Can you work these out from the model? Positions are in its coordinate system, mm. A direction names the side the tool comes from. Give positions to 0.01 mm unless a question says otherwise; leave off trailing zeros. Write each loop counter-clockwise with the first axis right and the second up, starting at its lowest first coordinate (ties: lowest second). Pieces come first, ordered by that corner, then holes.
1. I'm going to push flat-ended pins straight in: pin 1 (0.8 mm diameter, centred on x = 27.5, z = 14.5, fed in from -Y); pin 2 (8 mm diameter, centred on y = 25, z = 2.5, fed in from -X); pin 3 (1.5 mm diameter, centred on y = 3, z = 9.5, fed in from +X); pin 4 (3 mm diameter, centred on y = -14.5, z = 2, fed in from -X). Where does each tip first touch, or does it pass through?
2. Suppose I cut it at D-D (y = 3.5). Please give me the cut outline in (x, z), and give its area (3 significant figures).
3. Thinking about a two-plate mould opening in Y: for faces 1 (the flat face through (1, 59, 16)), 2 (the flat face through (8, -33.28, 3)), 3 (the flat face through (27, 1.8, 7.6)), which applies, pulls with the +Y half, pulls with the -Y half, needs draft (parallel to the pull), parting line crosses it, or undercut?
4. On a 3-axis mill with a long thin cutter (end or side, diameter ignored), from which of +Z, -Z, +X, -X, +Y, -Y can I reach the whole of each face in a straight line? I mean faces 4 (the flat face through (0, -21, 3)), 5 (the flat face through (0, 26, 3)), 6 (the flat face through (0, 59, 11)). Say none if no direction works.
5. Suppose I cut it at B-B (x = 20.5). Please give me the cut outline in (y, z), and give its area (3 significant figures).
6. Suppose I cut it at A-A (y = -18.5). Please give me the cut outline in (x, z), and give its area (3 significant figures).
7. Suppose I cut it at C-C (x = -5). Please give me the cut outline in (y, z).
8. If I drill on probe 1 along Y at (x, z) = (1, 4); probe 2 along X at (y, z) = (-3, 8.5); probe 3 along X at (y, z) = (-12.5, 5), over which ranges is the centre line in solid material (lowest first)?
```python
from build123d import *
from build123d import SkipClean  # not in build123d's __all__

# Parameters (mm, degrees)
F1_DEPTH  = 6
F3_DEPTH  = 10
F5_DEPTH  = 1
F7_DEPTH  = 1
F9_DEPTH  = 1
F10_DEPTH = 1
F13_DEPTH = 1


# Not quite as in the source:
# - ends of sketch curves that miss each other by under 0.0002 mm in the source are joined


with BuildPart() as f1:
    # F0 (on Top) → F1 (new body)
    with BuildSketch(Plane.XY):
        Polygon((-60, -8.2803227458), (-60, -33.2803227458), (-44, -33.2803227458), (-44, -8.2803227458), (0, -8.2803227458), (0, -33.2803227458), (16, -33.2803227458), (16, -8.2803227458), (28, -8.2803227458), (28, 11.7196772542), (0, 11.7196772542), (0, 40.7196772542), (28, 40.7196772542), (28, 60.7196772542), (-72, 60.7196772542), (-72, 40.7196772542), (-49, 40.7196772542), (-49, 11.7196772542), (-72, 11.7391310632), (-72, 11.693589665), (-72, 7.693589665), (-72, -4.280322887), (-72, -8.280322887), (-69, -8.2803227458), align=None)
    extrude(amount=F1_DEPTH)

    # F2 (on face) → F3 (join)
    with BuildSketch(Plane.XY.offset(6)):
        Polygon((-72, 60.7196772542), (-72, 56.7391310632), (-71, 56.7391310632), (-71, 58.7391310632), (-69, 58.7391310632), (-69, 60.7196772542), align=None)
        Polygon((-72, 40.7196773953), (-69, 40.7196773953), (-69, 42.7196773953), (-71, 42.7196773953), (-71, 44.7196773953), (-72, 44.7196773953), align=None)
        Polygon((-45, 42.7196773953), (-47, 42.7196773953), (-47, 40.7196773953), (-44, 40.7196773953), (-44, 44.7196773953), (-45, 44.7196773953), align=None)
        Polygon((-44, 60.7196772542), (-47, 60.7196772542), (-47, 58.7391310632), (-45, 58.7391310632), (-45, 56.7391310632), (-44, 56.7391310632), align=None)
        Polygon((28, 60.7196772542), (25, 60.7196772542), (25, 58.7391310632), (27, 58.7391310632), (27, 56.7391310632), (28, 56.7391310632), align=None)
        Polygon((25, 42.7196773953), (25, 40.7196773953), (28, 40.7196773953), (28, 44.7196773953), (27, 44.7196773953), (27, 42.7196773953), align=None)
        Polygon((0, 44.7196773953), (0, 40.7196772542), (3, 40.7196773953), (3, 42.7196773953), (1, 42.7196773953), (1, 44.7196773953), align=None)
        Polygon((3, 60.7196772542), (0, 60.7196772542), (0, 56.7391310632), (1, 56.7391310632), (1, 58.7391310632), (3, 58.7391310632), align=None)
        Polygon((27, 7.7391309221), (28, 7.7391309221), (28, 11.7196772542), (25, 11.7196772542), (25, 9.7391309221), (27, 9.7391309221), align=None)
        Polygon((25, -6.2803227458), (25, -8.2803227458), (28, -8.2803227458), (28, -4.2803227458), (27, -4.2803227458), (27, -6.2803227458), align=None)
        Polygon((0, -4.2803227458), (0, -8.280322887), (3, -8.2803227458), (3, -6.2803227458), (1, -6.2803227458), (1, -4.2803227458), align=None)
        Polygon((3, 9.7391309221), (3, 11.7196772542), (0, 11.7196772542), (0, 7.7391309221), (1, 7.7391309221), (1, 9.7391309221), align=None)
        Polygon((-45, 7.7391309221), (-44, 7.7391309221), (-44, 11.7391310632), (-47, 11.7391309221), (-47, 9.7391309221), (-45, 9.7391309221), align=None)
        Polygon((-47, -8.2803227458), (-44, -8.2803227458), (-44, -4.2803227458), (-45, -4.2803227458), (-45, -6.2803227458), (-47, -6.2803227458), align=None)
        Polygon((-72, -4.2803227458), (-72, -8.280322887), (-69, -8.2803227458), (-69, -6.2803227458), (-71, -6.2803227458), (-71, -4.2803227458), align=None)
        Polygon((-72, 11.7391310632), (-72, 7.7391309221), (-71, 7.7391309221), (-71, 9.7391309221), (-69, 9.7391309221), (-69, 11.7365936099), align=None)
    with SkipClean():  # cleaning this boolean's faces spoils the solid; the shape is the same uncleaned
        extrude(amount=F3_DEPTH)

    # F4 (on face) → F5 (join)
    with BuildSketch(Plane.YZ.offset(28)):
        with BuildLine():
            ThreePointArc((7.7391309221, 13.6681435205), (1.7294040881, 7.8220547277), (-4.2803227458, 13.6681435205))
            Line((-4.2803227458, 13.6681435205), (-4.2803227458, 6))
            Line((-4.2803227458, 6), (7.7391309221, 6))
            Line((7.7391309221, 6), (7.7391309221, 13.6681435205))
        make_face()
    with SkipClean():  # cleaning this boolean's faces spoils the solid; the shape is the same uncleaned
        extrude(amount=-F5_DEPTH)

    # F6 (on face) → F7 (join)
    with BuildSketch(Plane.YZ.offset(28)):
        with BuildLine():
            ThreePointArc((56.7391310632, 13.6693800888), (50.7294042293, 7.8226900444), (44.7196773953, 13.6693800888))
            Line((44.7196773953, 13.6693800888), (44.7196773953, 6))
            Line((44.7196773953, 6), (56.7391310632, 6))
            Line((56.7391310632, 6), (56.7391310632, 13.6693800888))
        make_face()
    with SkipClean():  # cleaning this boolean's faces spoils the solid; the shape is the same uncleaned
        extrude(amount=-F7_DEPTH)

    # F8 (on face) → F9 (join)
    with BuildSketch(Plane(origin=(-72, 0, 0), x_dir=(0, -1, 0), z_dir=(-1, 0, 0))):
        with BuildLine():
            ThreePointArc((-44.7196773953, 14), (-50.7294042293, 8.1363701718), (-56.7391310632, 14))
            Line((-56.7391310632, 14), (-56.7391310632, 6))
            Line((-56.7391310632, 6), (-44.7196773953, 6))
            Line((-44.7196773953, 6), (-44.7196773953, 14))
        make_face()
    with SkipClean():  # cleaning this boolean's faces spoils the solid; the shape is the same uncleaned
        extrude(amount=-F9_DEPTH)

    # F12 (on face) → F13 (join)
    with BuildSketch(Plane(origin=(-72, 0, 0), x_dir=(0, -1, 0), z_dir=(-1, 0, 0))):
        with BuildLine():
            ThreePointArc((4.2803227458, 14), (-1.7294040881, 8.1533099556), (-7.7391309221, 14))
            Line((-7.7391309221, 14), (-7.7391309221, 6))
            Line((-7.7391309221, 6), (4.2803227458, 6))
            Line((4.2803227458, 6), (4.2803227458, 14))
        make_face()
    with SkipClean():  # cleaning this boolean's faces spoils the solid; the shape is the same uncleaned
        extrude(amount=-F13_DEPTH)


with BuildPart() as f10:
    # F8 (on face) → F10 (new body)
    with BuildSketch(Plane(origin=(-72, 0, 0), x_dir=(0, -1, 0), z_dir=(-1, 0, 0))):
        with BuildLine():
            ThreePointArc((4.282593064, 13.8288382557), (-1.649666924, 7.8232188447), (-7.7391309221, 13.6693800888))
            Line((-7.7391309221, 13.6693800888), (-7.7391309221, 5.9489118867))
            Line((-7.7391309221, 5.9489118867), (4.3871137314, 5.9489118867))
            Line((4.3871137314, 5.9489118867), (4.282593064, 13.8288382557))
        make_face()
    extrude(amount=-F10_DEPTH)


solid = f1.part
```
Checks:
1. pin 1: stops at y = -8.28
1. pin 2: stops at x = -49
1. pin 3: passes through
1. pin 4: stops at x = -60
2. outline: (-72, 0) - (28, 0) - (28, 8.09) - (27, 8.09) - (27, 6) - (-71, 6) - (-71, 8.42) - (-72, 8.42) - close
2. area: 605 mm2
3. face 1: needs draft
3. face 2: pulls with the -Y half
3. face 3: undercut
4. face 4: +Z, -Z, -Y
4. face 5: +Z, -Z, +X
4. face 6: +Z, +Y, -Y
5. outline: (-8.28, 0) - (11.72, 0) - (11.72, 6) - (-8.28, 6) - close; (40.72, 0) - (60.72, 0) - (60.72, 6) - (40.72, 6) - close
5. area: 240 mm2
6. outline: (-60, 0) - (-44, 0) - (-44, 6) - (-60, 6) - close; (0, 0) - (16, 0) - (16, 6) - (0, 6) - close
6. area: 192 mm2
7. outline: (-8.28, 0) - (60.72, 0) - (60.72, 6) - (-8.28, 6) - close
8. probe 1: y = -33.28 to 11.72, 40.72 to 60.72
8. probe 2: x = -72 to -71, 27 to 28
8. probe 3: x = -60 to -44, 0 to 16
